The listing builds one solid part. Answer for the finished solid, in the listing's coordinates (mm). A direction names the side the tool comes from. Give positions to 0.01 mm unless a question says otherwise; leave off trailing zeros. Write each loop counter-clockwise with the first axis right and the second up, starting at its lowest first coordinate (ties: lowest second). Pieces come first, ordered by that corner, then holes. Notation, with made-up numbers: (17.5, 71.25) - (73.5, 71.25) arc R23 cw to (73.5, 98.25) - close; hole circle Ø8 at (-26.5, -35.5). An arc over 180 degrees is marked (long way). One line per question, with ' | ' between items. Start each with the question number.
1. A cutting plane is placed at C-C (y = 0). Determine the outline of the cut face in (x, z).
2. A cutting plane is placed at D-D (x = 7). Determine the outline of the cut face in (y, z), then the cut area to 3 significant figures.
3. A cutting plane is placed at A-A (z = 15). Determine the outline of the cut face in (x, y).
4. Given P1, Ø4, axis at y = -6.5, z = -24, coming from the -X side; P2, Ø4, axis at x = -0.5, y = -1, coming from the +Z side; P3, Ø3, axis at y = -6.5, z = 4, coming from the +X side, each flat-ended and moving along its own axis, determine where each tip first touches the part or whether it passes through.
5. Find the intervals of material crossed by L1, parallel to X at y = -5.65, z = 15; L2, parallel to Z at x = 0, y = 6.05; L3, parallel to Z at x = -6.5, y = 2.5, in increasing order. Write a range as from..to.
6. A cutting plane is placed at B-B (x = 0). Determine the outline of the cut face in (y, z).
7. The mould has two halves that part along X. Classify faces 1 (the face through (-6, 0, -20)), 2 (the face through (0, -6, 12)), 3 (the face through (0, 8, 8)): +X half, -X half, draft (parallel to the pull), parting line (faces both ways), or undercut.
8. For faces 4 (the face through (-0.1, 7, 18.3)), 5 (the face through (-0.1, -7, 18.3)), 6 (the face through (0, -6, 25)), 7 (the face through (0, 0, 5)), 8 (the face through (2, 6, 0)), determine the directions among +Z, -Z, +X, -X, +Y, -Y from which every point of the face is accessible in a straight line to the end or side of a thin tool.
```python
from build123d import *

# Parameters (mm, degrees)
SZKIC1_W                        = 6
SZKIC1_H                        = 40
SZKIC2_W                        = 18
SZKIC2_H                        = 8
WYTNIJ_WYCI_GNI_CIE1_DEPTH      = 20
WYTNIJ_WYCI_GNI_CIE2_DEPTH      = 42.976183724
WYTNIJ_WYCI_GNI_CIE2_DEPTH_BACK = 42.976183724
SZKIC3_R                        = 3
WYTNIJ_WYCI_GNI_CIE3_START      = 7
SZKIC3_4_W                      = 16.124515496
SZKIC3_4_H                      = 17
SZKIC3_4_R                      = 3
WYTNIJ_WYCI_GNI_CIE3_DEPTH      = 35.976183767


with BuildPart() as part:
    # Szkic1 → Obr_t1 (revolve)
    with BuildSketch(Plane(origin=(0, 0, 0), x_dir=(1, 0, 0), z_dir=(0, 1, 0))):
        with Locations((3, 20)):
            Rectangle(SZKIC1_W, SZKIC1_H)
        Polygon((0, 0), (0, -25), (9, -25), (9, 0), (6, 0), align=None)
    revolve(axis=Axis((0, 0, 44.409951059), (0, 0, -1)))

    # Szkic2 → Wytnij-wyci_gni_cie1 (cut)
    with BuildSketch(Plane.XY.offset(25)):
        Rectangle(SZKIC2_W, SZKIC2_H)
    extrude(amount=-WYTNIJ_WYCI_GNI_CIE1_DEPTH, mode=Mode.SUBTRACT)

    # Szkic3 → Wytnij-wyci_gni_cie2 (cut, two sides: drawn at the far end of the back side and taken through both)
    with BuildSketch(Plane(origin=(0, 0, 0), x_dir=(1, 0, 0), z_dir=(0, 1, 0)).offset(-WYTNIJ_WYCI_GNI_CIE2_DEPTH_BACK)):
        with Locations(Location((0, -15, 0), (0, 0, 270))):
            Circle(SZKIC3_R)
    extrude(amount=WYTNIJ_WYCI_GNI_CIE2_DEPTH + WYTNIJ_WYCI_GNI_CIE2_DEPTH_BACK, mode=Mode.SUBTRACT)

    # Szkic3_4 → Wytnij-wyci_gni_cie3 (cut, through all)
    with BuildSketch(Plane(origin=(0, 0, 0), x_dir=(1, 0, 0), z_dir=(0, 1, 0)).offset(WYTNIJ_WYCI_GNI_CIE3_START)):
        with Locations((0, -16.5)):
            Rectangle(SZKIC3_4_W, SZKIC3_4_H)
        with Locations(Location((0, -15, 0), (0, 0, 270))):
            Circle(SZKIC3_4_R, mode=Mode.SUBTRACT)
    wytnij_wyci_gni_cie3 = extrude(amount=WYTNIJ_WYCI_GNI_CIE3_DEPTH, mode=Mode.SUBTRACT)

    # Lustro1: Wytnij-wyci_gni_cie3 across plane
    add(wytnij_wyci_gni_cie3.mirror(Plane.ZX), mode=Mode.SUBTRACT)


solid = part.part
```
Determined:
1) outline: (-9, 0) - (-6, 0) - (-6, -40) - (6, -40) - (6, 0) - (9, 0) - (9, 5) - (-9, 5) - close
2) outline: (-5.66, 0) - (5.66, 0) - (5.66, 25) - (4, 25) - (4, 5) - (-4, 5) - (-4, 25) - (-5.66, 25) - close | area: 123 mm2
3) outline: (-8.06, -4) arc R9 ccw to (-5.66, -7) - (-3, -7) - (-3, -4) - close; (-8.06, 4) - (-3, 4) - (-3, 7) - (-5.66, 7) arc R9 ccw to start; (3, -7) - (5.66, -7) arc R9 ccw to (8.06, -4) - (3, -4) - close; (3, 4) - (8.06, 4) arc R9 ccw to (5.66, 7) - (3, 7) - close
4) P1: x = -3.97 | P2: z = 5 | P3: x = 7.48
5) L1: -7.01..-3, 3..7.01 | L2: 0..12, 18..25 | L3: 0..5
6) outline: (-9, 0) - (-6, 0) - (-6, -40) - (6, -40) - (6, 0) - (9, 0) - (9, 8) - (7, 8) - (7, 12) - (4, 12) - (4, 5) - (-4, 5) - (-4, 12) - (-7, 12) - (-7, 8) - (-9, 8) - close; (-7, 18) - (-4, 18) - (-4, 25) - (-7, 25) - close; (4, 18) - (7, 18) - (7, 25) - (4, 25) - close
7) face 1: parting line | face 2: undercut | face 3: draft
8) face 4: +Z, +X, -X, +Y | face 5: +Z, +X, -X, -Y | face 6: +Z, +X, -X, +Y, -Y | face 7: +Z, +X, -X | face 8: -Z
